For this review, use the dimensioned drawing (mm, ordinates from the lowest corner) and the shaded views. A direction names the side the tool comes from. Give positions to 0.01 mm unless a question says otherwise; leave off trailing zeros. Order: outer loops, then holes, each group sorted by start corner. A loop starts at its lowest first (then second) coordinate and runs counter-clockwise, first axis right, second up.
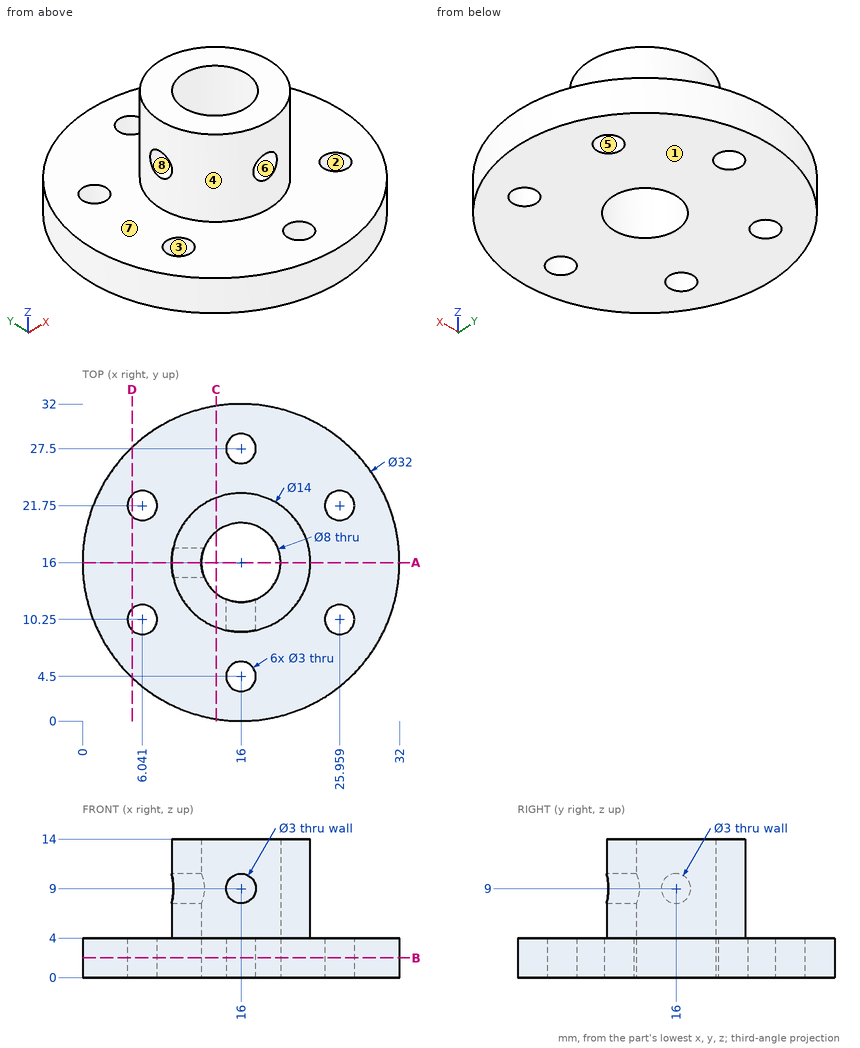
1. Insertion check: pin 1 (4 mm diameter, centred on x = 25.96, y = 10.25, fed in from -Z); pin 2 (1.5 mm diameter, centred on y = 21, z = 3, fed in from -X) (1 decimal); pin 3 (5 mm diameter, centred on x = 25.96, y = 21.75, fed in from +Z); pin 4 (3 mm diameter, centred on y = 19.5, z = 6.5, fed in from +X). Each pin has a flat end and moves straight along its axis. Give the tip position at first contact, or say it passes through.
2. Take a section at B-B (z = 2). Write out the cut boundary in (x, y).
3. For the marked faces 5, 6, 7 and 8, list the 3-axis set-ups (+Z, -Z, +X, -X, +Y, -Y) from which the entire face can be reached by the end or side of a thin tool; tool diameter is ignored.
4. To check wall thickness, follow line 1 (Y direction, x = 16, z = 0.95); line 2 (Z direction, x = 16, y = 10); line 3 (Z direction, x = 26, y = 8). State the ranges of each line that lie inside material, in increasing order.
5. Draft analysis for pull direction X (two halves, no side actions). For the marked faces 1, 2, 3 and 4, state which applies: pulls with the +X half, pulls with the -X half, needs draft (parallel to the pull), parting line crosses it, or undercut.
6. Take a section at D-D (x = 5). Write out the cut boundary in (y, z).
7. Take a section at C-C (x = 13.5). Write out the cut boundary in (y, z).
8. Take a section at A-A (y = 16). Write out the cut boundary in (x, z), and give its area (3 significant figures).
Answer:
1. pin 1: stops at z = 0
1. pin 2: stops at x = 0.6
1. pin 3: stops at z = 4
1. pin 4: stops at x = 22.71
2. outline: circle Ø32 at (16, 16); hole circle Ø3 at (6.04, 10.25); hole circle Ø3 at (6.04, 21.75); hole circle Ø8 at (16, 16); hole circle Ø3 at (16, 4.5); hole circle Ø3 at (16, 27.5); hole circle Ø3 at (25.96, 10.25); hole circle Ø3 at (25.96, 21.75)
3. face 5: +Z, -Z
3. face 6: -Y
3. face 7: +Z
3. face 8: -X
4. line 1: y = 0 to 3, 6 to 12, 20 to 26, 29 to 32
4. line 2: z = 0 to 7.5, 10.5 to 14
4. line 3: z = 0 to 4
5. face 1: needs draft
5. face 2: undercut
5. face 3: undercut
5. face 4: parting line crosses it
6. outline: (4.38, 0) - (9.17, 0) - (9.17, 4) - (4.38, 4) - close; (11.33, 0) - (20.67, 0) - (20.67, 4) - (11.33, 4) - close; (22.83, 0) - (27.62, 0) - (27.62, 4) - (22.83, 4) - close
7. outline: (0.2, 0) - (12.88, 0) - (12.88, 14) - (9.46, 14) - (9.46, 4) - (0.2, 4) - close; (19.12, 0) - (31.8, 0) - (31.8, 4) - (22.54, 4) - (22.54, 14) - (19.12, 14) - close
8. outline: (0, 0) - (12, 0) - (12, 7.5) - (9, 7.5) - (9, 4) - (0, 4) - close; (9, 10.5) - (12, 10.5) - (12, 14) - (9, 14) - close; (20, 0) - (32, 0) - (32, 4) - (23, 4) - (23, 14) - (20, 14) - close
8. area: 147 mm2
